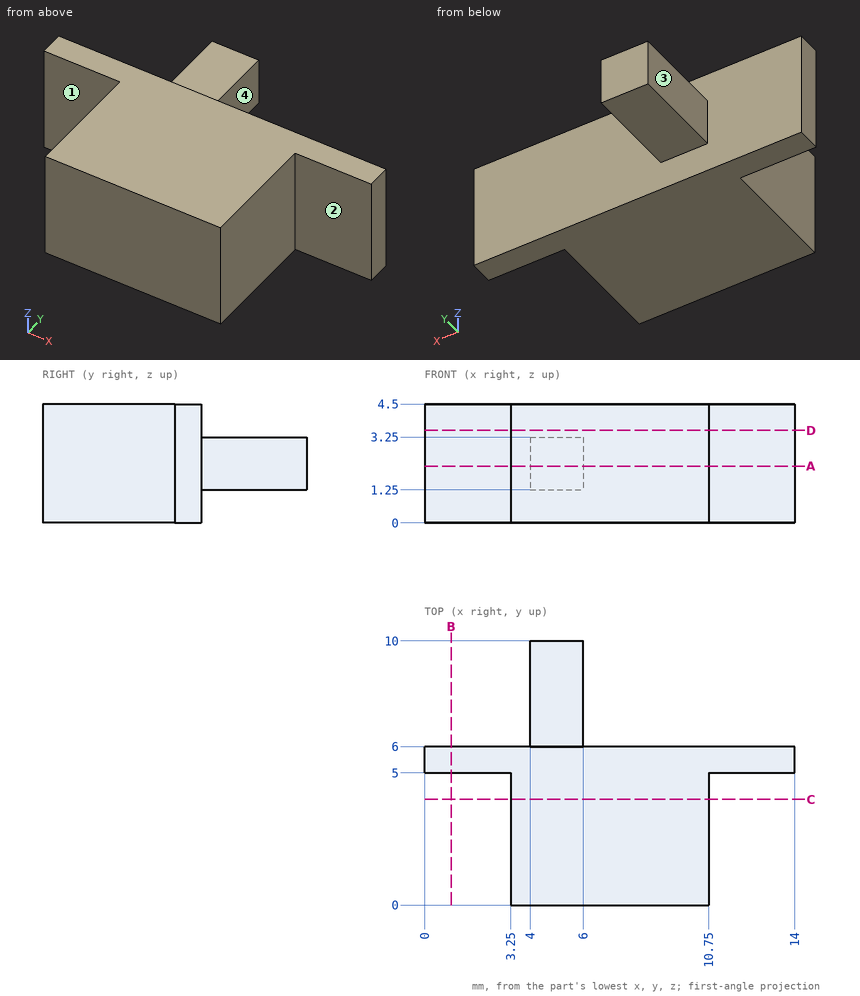
For this review, use the dimensioned drawing (mm, ordinates from the lowest corner) and the shaded views. A direction names the side the tool comes from. Coordinates: 2 decimals unless noted, no trailing zeros. Write each loop counter-clockwise with the first axis right and the second up, starting at its lowest first coordinate (ties: lowest second). Pieces come first, ordered by that corner, then holes. Notation, with made-up numbers: (11, -8) -> (50, -8) arc R15 ccw to (50, -4) -> close; hole circle Ø11 at (-11.75, 49.5). An arc over 180 degrees is marked (long way). Put each result on its own line as item: value.
Q1. Clearance check with flat-ended pins moving along their axes: pin 1 Ø2 at (y, z) = (8.5, 2.5) entering from -X; pin 2 Ø1.6 at (y, z) = (7, 2) entering from +X; pin 3 Ø2.5 at (x, z) = (1, 1.5) entering from -Y; pin 4 Ø3 at (x, y) = (2.5, 1.5) entering from -Z. State where each tip first meets the part, or that it passes through.
From the geometry:
pin 1: stops at x = 4
pin 2: stops at x = 6
pin 3: stops at y = 5
pin 4: stops at z = 0
Q2. Wall thickness on L1, parallel to Y at x = 12, z = 1.65; L2, parallel to X at y = 6.75, z = 2.3; L3, parallel to Y at x = 7.5, z = 2.3: over which ranges is each line inside the solid? List them lowest first.
From the geometry:
L1: y = 5 to 6
L2: x = 4 to 6
L3: y = 0 to 6
Q3. Take a section at C-C, the plane y = 4. State the section outline as (x, z) points, then the cut area to 4 significant figures.
From the geometry:
outline: (3.25, 0) -> (10.75, 0) -> (10.75, 4.5) -> (3.25, 4.5) -> close
area: 33.75 mm2
Q4. Tool access review of the marked faces 1, 2, 3 and 4: name each direction out of +Z, -Z, +X, -X, +Y, -Y from which nothing blocks a thin tool from reaching the whole face with its end or side.
From the geometry:
face 1: +Z, -Z, -X, -Y
face 2: +Z, -Z, +X, -Y
face 3: +Z, -Z, -X, +Y
face 4: +Z, -Z, +X, +Y
Q5. Take a section at B-B, the plane x = 1. State the section outline as (y, z) points.
From the geometry:
outline: (5, 0) -> (6, 0) -> (6, 4.5) -> (5, 4.5) -> close
Q6. Take a section at D-D, the plane z = 3.5. State the section outline as (x, y) points, then the cut area to 3 significant figures.
From the geometry:
outline: (0, 5) -> (3.25, 5) -> (3.25, 0) -> (10.75, 0) -> (10.75, 5) -> (14, 5) -> (14, 6) -> (0, 6) -> close
area: 51.5 mm2
Q7. Take a section at A-A, the plane z = 2.15. State the section outline as (x, y) points, then the cut area to 3 significant figures.
From the geometry:
outline: (0, 5) -> (3.25, 5) -> (3.25, 0) -> (10.75, 0) -> (10.75, 5) -> (14, 5) -> (14, 6) -> (6, 6) -> (6, 10) -> (4, 10) -> (4, 6) -> (0, 6) -> close
area: 59.5 mm2
